For this review, take the finished solid that the model builds, in its own axes (mm). A direction names the side the tool comes from. Round coordinates to 2 decimals unless told otherwise and drop trailing zeros. Loops run counter-clockwise (first coordinate to the right, second up) from the corner with the lowest first, then second, coordinate; pieces in that order, holes last.
1) Take a section at D-D (y = 47). Give the number of separate pieces and of enclosed holes in the cut face, then the cut area to 3 significant figures.
2) Take a section at B-B (x = -95.25). State the section outline as (y, z) points (3 decimals).
3) Take a section at C-C (x = -19.05). State the section outline as (y, z) points (3 decimals), then the cut area to 3 significant figures.
4) Wall thickness on L1, parallel to Y at x = -6.35, z = 7; L2, parallel to X at y = 39, z = 5; L3, parallel to X at y = 6.5, z = 9: over which ranges is each line inside the solid? List them lowest first.
5) Insertion check: pin 1 (1.5 mm diameter, centred on y = 37.5, z = 3.5, fed in from +X); pin 2 (2.5 mm diameter, centred on x = -6.35, y = 44.45, fed in from -Z). Each pin has a flat end and moves straight along its axis. Give the tip position at first contact, or say it passes through.
6) Take a section at A-A (y = 6.35). State the section outline as (x, z) points (3 decimals), then the cut area to 3 significant figures.
7) Tool access review of faces 4 (the cylindrical face through (-43.177, 40.966, 3.595)), 5 (the flat face through (-52, 26, 9.525)): name each direction out of +Z, -Z, +X, -X, +Y, -Y from which nothing blocks a thin tool from reaching the whole face with its end or side.
8) Mouldability with a two-part tool opening along Y and no side actions: class faces 1 (the flat face through (-52, 50.8, 5)), 2 (the flat face through (0, 25, 5)), 3 (the cylindrical face through (-84.058, 12.075, 4.696)) as pulls with the +Y half, pulls with the -Y half, needs draft (parallel to the pull), parting line crosses it, or undercut.
```python
from build123d import *

# Parameters (mm, degrees)
SKETCH1_W                       = 101.6
SKETCH1_H                       = 50.8
BOSS_EXTRUDE1_DEPTH             = 9.525
F_8_32_TAPPED_HOLE1_D           = 3.4544
F_8_32_TAPPED_HOLE1_DEPTH       = 19.05
F_8_32_TAPPED_HOLE1_CSINK_D     = 4.1656
F_8_32_TAPPED_HOLE1_CSINK_ANGLE = 90
F_8_32_TAPPED_HOLE1_TIP         = 1.037806461
F_4_CLEARANCE_HOLE2_D           = 3.2639
F_4_CLEARANCE_HOLE2_DEPTH       = 25.4
F_4_CLEARANCE_HOLE2_TIP         = 0.980574487
F_6_32_TAPPED_HOLE1_D           = 2.7051
F_4_CLEARANCE_HOLE1_D           = 3.2639
F_4_CLEARANCE_HOLE1_DEPTH       = 9.525


with BuildPart() as part:
    # Sketch1 → Boss-Extrude1 (new body)
    with BuildSketch(Plane.XY):
        with Locations((-50.8, 25.4)):
            Rectangle(SKETCH1_W, SKETCH1_H)
    extrude(amount=BOSS_EXTRUDE1_DEPTH)

    # #8-32 Tapped Hole1
    with Locations(Plane(origin=(0, 50.8, 0), x_dir=(1, 0, 0), z_dir=(0, 1, 0))):
        with Locations((-44.45, -4.7625), (-57.15, -4.7625)):
            CounterSinkHole(F_8_32_TAPPED_HOLE1_D / 2, F_8_32_TAPPED_HOLE1_CSINK_D / 2, depth=F_8_32_TAPPED_HOLE1_DEPTH, counter_sink_angle=F_8_32_TAPPED_HOLE1_CSINK_ANGLE)
            with Locations((0, 0, -(F_8_32_TAPPED_HOLE1_DEPTH + F_8_32_TAPPED_HOLE1_TIP / 2))):  # 118° drill point
                Cone(0, F_8_32_TAPPED_HOLE1_D / 2, F_8_32_TAPPED_HOLE1_TIP, mode=Mode.SUBTRACT)

    # #4 Clearance Hole2
    with Locations(Plane.XY.offset(9.525)):
        with Locations((-44.45, 30.712193539), (-57.15, 30.712193539)):
            Hole(F_4_CLEARANCE_HOLE2_D / 2, depth=F_4_CLEARANCE_HOLE2_DEPTH)
            with Locations((0, 0, -(F_4_CLEARANCE_HOLE2_DEPTH + F_4_CLEARANCE_HOLE2_TIP / 2))):  # 118° drill point
                Cone(0, F_4_CLEARANCE_HOLE2_D / 2, F_4_CLEARANCE_HOLE2_TIP, mode=Mode.SUBTRACT)

    # #6-32 Tapped Hole1 (through all)
    with Locations(Plane.XY.offset(9.525)):
        with Locations((-95.25, 6.35), (-95.25, 44.45), (-6.35, 6.35), (-6.35, 44.45)):
            Hole(F_6_32_TAPPED_HOLE1_D / 2)

    # #4 Clearance Hole1
    with Locations(Plane.XY.offset(9.525)):
        with Locations((-82.55, 12.7), (-19.05, 12.7)):
            Hole(F_4_CLEARANCE_HOLE1_D / 2, depth=F_4_CLEARANCE_HOLE1_DEPTH)


solid = part.part
```
Response:
1. separate pieces: 1
1. enclosed holes: 2
1. area: 949 mm2
2. outline: (0, 0) - (4.997, 0) - (4.997, 9.525) - (0, 9.525) - close; (7.703, 0) - (43.097, 0) - (43.097, 9.525) - (7.703, 9.525) - close; (45.803, 0) - (50.8, 0) - (50.8, 9.525) - (45.803, 9.525) - close
3. outline: (0, 0) - (11.068, 0) - (11.068, 9.525) - (0, 9.525) - close; (14.332, 0) - (50.8, 0) - (50.8, 9.525) - (14.332, 9.525) - close
3. area: 453 mm2
4. L1: y = 0 to 5, 7.7 to 43.1, 45.8 to 50.8
4. L2: x = -101.6 to -58.86, -55.44 to -46.16, -42.74 to 0
4. L3: x = -101.6 to -96.59, -93.91 to -7.69, -5.01 to 0
5. pin 1: stops at x = 0
5. pin 2: passes through
6. outline: (-101.6, 0) - (-96.603, 0) - (-96.603, 9.525) - (-101.6, 9.525) - close; (-93.897, 0) - (-7.703, 0) - (-7.703, 9.525) - (-93.897, 9.525) - close; (-4.997, 0) - (0, 0) - (0, 9.525) - (-4.997, 9.525) - close
6. area: 916 mm2
7. face 4: +Y
7. face 5: +Z, +X, -X, +Y, -Y
8. face 1: pulls with the +Y half
8. face 2: needs draft
8. face 3: undercut
